Verification items for the finished model (mm, model axes). A direction names the side the tool comes from. Round coordinates to 2 decimals unless told otherwise and drop trailing zeros. Write each loop counter-clockwise with the first axis right and the second up, starting at its lowest first coordinate (ties: lowest second). Pieces come first, ordered by that corner, then holes. Notation, with made-up numbers: (80, 33.5) - (132, 33.5) arc R29 cw to (132, 71.5) - close; hole circle Ø9 at (29.25, 69.5). An arc over 180 degrees is marked (long way). Answer as a JSON object with one key per item and string values.
```python
from build123d import *

# Parameters (mm, degrees)
SKETCH_1_W           = 32
SKETCH_1_H           = 42.5
EXTRUDE_1_DEPTH      = 3
EXTRUDE_2_DEPTH      = 3
EXTRUDE_2_DEPTH_BACK = 35
SKETCH_2_W           = 3
SKETCH_2_H           = 20
CUT_EXTRUDE_1_DEPTH  = 3
SKETCH_4_W           = 5
SKETCH_4_H           = 9
CUT_EXTRUDE_2_DEPTH  = 3


with BuildPart() as part:
    # Sketch 1 → Extrude 1 (new body)
    with BuildSketch(Plane.XY):
        with Locations((16, 21.25)):
            Rectangle(SKETCH_1_W, SKETCH_1_H)
    extrude(amount=EXTRUDE_1_DEPTH)

    # Sketch 2 → Extrude 2 (add, two sides: drawn at the far end of the back side and taken through both)
    with BuildSketch(Plane(origin=(32, 0, 0), x_dir=(0, 0, -1), z_dir=(1, 0, 0)).offset(-EXTRUDE_2_DEPTH_BACK)):
        with Locations((-1.5, 13.5)):
            Rectangle(SKETCH_2_W, SKETCH_2_H)
    extrude(amount=EXTRUDE_2_DEPTH + EXTRUDE_2_DEPTH_BACK)

    # Sketch 3 → Cut-Extrude 1 (cut)
    with BuildSketch(Plane.XY.offset(3)):
        Polygon((14.5, 42.5), (14.5, 36.5), (13.25, 36.5), (13.25, 34), (14.5, 34), (14.5, 28), (17.5, 28), (17.5, 34), (18.75, 34), (18.75, 36.5), (17.5, 36.5), (17.5, 42.5), align=None)
    extrude(amount=-CUT_EXTRUDE_1_DEPTH, mode=Mode.SUBTRACT)

    # Sketch 4 → Cut-Extrude 2 (cut)
    with BuildSketch(Plane.XY.offset(3)):
        with Locations((2.5, 38)):
            Rectangle(SKETCH_4_W, SKETCH_4_H)
    extrude(amount=-CUT_EXTRUDE_2_DEPTH, mode=Mode.SUBTRACT)


solid = part.part
```
1. Cross-section at D-D (x = 4). Record the boundary of the cut face in (y, z).
Completed:
{"outline": "(0, 0) - (33.5, 0) - (33.5, 3) - (0, 3) - close"}
2. Cross-section at C-C (y = 35.5). Record the boundary of the cut face in (x, z), plus the area to 3 significant figures.
Completed:
{"outline": "(5, 0) - (13.25, 0) - (13.25, 3) - (5, 3) - close; (18.75, 0) - (32, 0) - (32, 3) - (18.75, 3) - close", "area": "64.5 mm^2"}
3. Mould release check, pull along X, two halves, no side actions. Record for faces 6 (the face through (2, 33.5, 2)), 7 (the face through (18, 34, 2)), 8 (the face through (5, 38, 2)): released by +X, released by -X, zero draft, split by the parting line, or undercut.
Completed:
{"face 6": "zero draft", "face 7": "undercut", "face 8": "released by -X"}
4. Access from +Z, -Z, +X, -X, +Y, -Y to the whole of each face (thin tool, end or side, straight path). Record for faces 1 (the face through (18, 36.5, 2)), 2 (the face through (33, 3.5, 2)), 3 (the face through (-2, 23.5, 2)), 4 (the face through (17.5, 39, 2)), 5 (the face through (-3, 14, 2)).
Completed:
{"face 1": "+Z, -Z", "face 2": "+Z, -Z, +X, -Y", "face 3": "+Z, -Z, -X, +Y", "face 4": "+Z, -Z, +Y", "face 5": "+Z, -Z, -X, +Y, -Y"}
5. Cross-section at A-A (y = 30). Record the boundary of the cut face in (x, z).
Completed:
{"outline": "(0, 0) - (14.5, 0) - (14.5, 3) - (0, 3) - close; (17.5, 0) - (32, 0) - (32, 3) - (17.5, 3) - close"}
6. Cross-section at B-B (z = 0.8). Record the boundary of the cut face in (x, y), plus the area to 3 significant figures.
Completed:
{"outline": "(-3, 3.5) - (0, 3.5) - (0, 0) - (32, 0) - (32, 3.5) - (35, 3.5) - (35, 23.5) - (32, 23.5) - (32, 42.5) - (17.5, 42.5) - (17.5, 36.5) - (18.75, 36.5) - (18.75, 34) - (17.5, 34) - (17.5, 28) - (14.5, 28) - (14.5, 34) - (13.25, 34) - (13.25, 36.5) - (14.5, 36.5) - (14.5, 42.5) - (5, 42.5) - (5, 33.5) - (0, 33.5) - (0, 23.5) - (-3, 23.5) - close", "area": "1,390 mm^2"}
7. Material ranges on probe 1 along Y at (x, z) = (13.5, 1.95); probe 2 along X at (y, z) = (35.5, 2.5); probe 3 along X at (y, z) = (41, 1.85), recorded low to high. Write a range as from..to.
Completed:
{"probe 1": "y = 0..34, 36.5..42.5", "probe 2": "x = 5..13.25, 18.75..32", "probe 3": "x = 5..14.5, 17.5..32"}
8. Go/stop test with flat-tipped pins: pin 1 (1.5 mm diameter, centred on y = 28.5, z = 2, fed in from +X); pin 2 (1.5 mm diameter, centred on y = 35.5, z = 2, fed in from -X); pin 3 (0.9 mm diameter, centred on y = 2, z = 2, fed in from -X). Record where each tip stops, or that it passes through.
Completed:
{"pin 1": "stops at x = 32", "pin 2": "stops at x = 5", "pin 3": "stops at x = 0"}
